Check sheet for the modelled part. Datum: model origin and axes. Units: mm. A direction names the side the tool comes from. Coordinates: 2 decimals unless noted, no trailing zeros. Write each loop counter-clockwise with the first axis right and the second up, starting at its lowest first coordinate (ties: lowest second). Pieces come first, ordered by that corner, then holes. Notation, with made-up numbers: (13, -19) - (38, -19) arc R5 cw to (38, -13) - close; hole circle Ø10 at (84.5, -38). An arc over 180 degrees is marked (long way). Answer as CSV lines item,"result". Start each with the question number.
from build123d import *

# Parameters (mm, degrees)
SKETCH1_R           = 6
BOSS_EXTRUDE1_DEPTH = 81.92
SKETCH3_R           = 3
BOSS_EXTRUDE2_DEPTH = 3.2
SKETCH4_W           = 6.3
SKETCH4_H           = 6.3
BOSS_EXTRUDE3_DEPTH = 3.25
SKETCH10_R          = 3
BOSS_EXTRUDE6_DEPTH = 1
BOSS_EXTRUDE7_DEPTH = 8.5
SKETCH12_R          = 5.645731703
SKETCH12_R_2        = 3.9
CUT_EXTRUDE2_DEPTH  = 2.2
SKETCH14_R          = 3.959834879
SKETCH14_R_2        = 2.65
CUT_EXTRUDE3_DEPTH  = 0.89


with BuildPart() as part:
    # Sketch1 → Boss-Extrude1 (new body)
    with BuildSketch(Plane.XY):
        Circle(SKETCH1_R)
    extrude(amount=BOSS_EXTRUDE1_DEPTH)

    # Sketch2 → Revolve1 (revolve)
    with BuildSketch(Plane(origin=(0, 0, 0), x_dir=(1, 0, 0), z_dir=(0, 1, 0))):
        Polygon((-1.987053294, 0), (-1.987053294, 1.5), (-3.1, 1.5), (-3.1, 6.3), (0, 6.3), (0, 0), align=None)
    revolve(axis=Axis((0, 0, 88.862708705), (0, 0, 1)))

    # Sketch3 → Boss-Extrude2 (add)
    with BuildSketch(Plane.XY.offset(81.92)):
        Circle(SKETCH3_R)
    extrude(amount=BOSS_EXTRUDE2_DEPTH)

    # Sketch4 → Boss-Extrude3 (add, symmetric)
    with BuildSketch(Plane(origin=(0, 0, 0), x_dir=(1, 0, 0), z_dir=(0, 1, 0))):
        with Locations((0, -88.27)):
            Rectangle(SKETCH4_W, SKETCH4_H)
    extrude(amount=BOSS_EXTRUDE3_DEPTH, both=True)

    # Sketch9 → Cut-Revolve3 (revolve, cut)
    with BuildSketch(Plane(origin=(0, 0, 0), x_dir=(1, 0, 0), z_dir=(0, 1, 0))):
        Polygon((-3.15, -91.42), (-4.65, -90.92), (-4.65, -91.42), align=None)
        Polygon((-3.15, -85.12), (-4.65, -85.12), (-4.65, -85.62), align=None)
    revolve(axis=Axis((0, 0, 97.04036036), (0, 0, -1)), mode=Mode.SUBTRACT)

    # Sketch10 → Boss-Extrude6 (add, symmetric)
    with BuildSketch(Plane(origin=(0, 3.25, 0), x_dir=(1, 0, 0), z_dir=(0, 1, 0))):
        with Locations((0, -88.27)):
            Circle(SKETCH10_R)
    extrude(amount=BOSS_EXTRUDE6_DEPTH, both=True)

    # Sketch11 → Boss-Extrude7 (add)
    with BuildSketch(Plane(origin=(0, 4.25, 0), x_dir=(1, 0, 0), z_dir=(0, 1, 0))):
        Polygon((0, -83.651197846), (-4, -85.960598923), (-4, -90.579401077), (0, -92.888802154), (4, -90.579401077), (4, -85.960598923), align=None)
    extrude(amount=BOSS_EXTRUDE7_DEPTH)

    # Sketch12 → Cut-Extrude2 (cut)
    with BuildSketch(Plane(origin=(0, 12.75, 0), x_dir=(1, 0, 0), z_dir=(0, 1, 0))):
        with Locations((0, -88.27)):
            Circle(SKETCH12_R)
        with Locations((0, -88.27)):
            Circle(SKETCH12_R_2, mode=Mode.SUBTRACT)
    extrude(amount=-CUT_EXTRUDE2_DEPTH, mode=Mode.SUBTRACT)

    # Sketch13 → Cut-Revolve4 (revolve, cut)
    with BuildSketch(Plane(origin=(0, 0, 0), x_dir=(0, 0, -1), z_dir=(1, 0, 0))):
        Polygon((-92.17, 10.55), (-92.888802154, 10.15), (-92.888802154, 10.55), align=None)
        Polygon((-92.888802154, 4.65), (-92.17, 4.25), (-92.888802154, 4.25), align=None)
    revolve(axis=Axis((0, 13.752185795, 88.27), (0, -1, 0)), mode=Mode.SUBTRACT)

    # Sketch14 → Cut-Extrude3 (cut)
    with BuildSketch(Plane(origin=(0, 0, -6.3), x_dir=(-1, 0, 0), z_dir=(0, 0, -1))):
        Circle(SKETCH14_R)
        Circle(SKETCH14_R_2, mode=Mode.SUBTRACT)
    extrude(amount=-CUT_EXTRUDE3_DEPTH, mode=Mode.SUBTRACT)


solid = part.part
(1) Release check for a two-part mould opening along Z. For faces 1 (the face through (-0.845, 11.665, 92.077)), 2 (the face through (-6, 0, 40)), 3 (the face through (-3, -1, 81.92)) record: pulls with the +Z half, pulls with the -Z half, needs draft (parallel to the pull), parting line crosses it, or undercut.
(2) Cross-section at C-C on z = 1. Record the boundary of the cut face in (x, y).
(3) Tool access check on faces 4 (the face through (-3, 0, 83)), 5 (the face through (3.15, 0, 88)), 6 (the face through (0, -3.25, 88)), 7 (the face through (-1.43, 2.75, -3.48)). Record the directions out of +Z, -Z, +X, -X, +Y, -Y that give a thin tool (end or side, any length) a straight path to the whole face; none if there is none.
(4) Material ranges on probe 1 along Z at (x, y) = (1.25, 2); probe 2 along Y at (x, z) = (0, 47); probe 3 along Z at (x, y) = (1.5, 0.75), recorded low to high. Write a range as from..to.
(5) Cross-section at B-B on y = 9.25. Record the boundary of the cut face in (x, z).
(6) Cross-section at D-D on y = -4.25. Record the boundary of the cut face in (x, z), plus the area to 3 significant figures.
(7) Go/stop test with flat-tipped pins: P1, Ø5, axis at x = -0.5, z = 89.5, coming from the -Y side; P2, Ø7, axis at y = 1.5, z = 87.5, coming from the +X side; P3, Ø7, axis at x = -0.5, y = -1, coming from the +Z side; P4, Ø8, axis at y = 3.5, z = 70, coming from the +X side. Record where each tip stops, or that it passes through.
(8) Cross-section at A-A on z = 88.27. Record the boundary of the cut face in (x, y).
Checked values:
1,face 1,"parting line crosses it"
1,face 2,"needs draft"
1,face 3,"undercut"
2,outline,"circle Ø12 at (0, 0)"
3,face 4,"none"
3,face 5,"+Z, +X, -Y"
3,face 6,"+Z, +X, -X, -Y"
3,face 7,"-Z"
4,probe 1,"-6.3..-1.5, 0..91.42"
4,probe 2,"-6..6"
4,probe 3,"-6.3..91.42"
5,outline,"(-4, 85.96) - (0, 83.65) - (4, 85.96) - (4, 90.58) - (0, 92.89) - (-4, 90.58) - close"
6,outline,"(-4.24, 0) - (4.24, 0) - (4.24, 81.92) - (-4.24, 81.92) - close"
6,area,"694 mm^2"
7,P1,"y = -3.25"
7,P2,"x = 4"
7,P3,"z = 91.42"
7,P4,"x = 6"
8,outline,"(-4, 4.31) - (-3.9, 4.25) - (-3, 4.25) - (-3, 3.25) - (-3.15, 3.25) - (-3.15, -3.25) - (3.15, -3.25) - (3.15, 3.25) - (3, 3.25) - (3, 4.25) - (3.9, 4.25) - (4, 4.31) - (4, 10.49) - (3.9, 10.55) - (3.9, 12.75) - (-3.9, 12.75) - (-3.9, 10.55) - (-4, 10.49) - close"
